```python
from build123d import *

# Parameters (mm, degrees)
SKETCH1_W           = 50.8
SKETCH1_H           = 50.8
BOSS_EXTRUDE1_DEPTH = 1.5875
SKETCH3_R           = 1.2065
BOSS_EXTRUDE2_DEPTH = 8.89
SKETCH4_R           = 2.54
SKETCH4_R_2         = 1.27
CUT_EXTRUDE1_DEPTH  = 43.790708396
BOSS_EXTRUDE3_START = 12.065
SKETCH5_R           = 1.2065
BOSS_EXTRUDE3_DEPTH = 12.065


with BuildPart() as part:
    # Sketch1 → Boss-Extrude1 (new, symmetric)
    with BuildSketch(Plane(origin=(0, 0, 0), x_dir=(1, 0, 0), z_dir=(0, 1, 0))):
        Rectangle(SKETCH1_W, SKETCH1_H)
    extrude(amount=BOSS_EXTRUDE1_DEPTH, both=True)

    # Sketch3 → Boss-Extrude2 (add)
    with BuildSketch(Plane(origin=(25.4, 0, 0), x_dir=(0, 0, -1), z_dir=(1, 0, 0))):
        with Locations(Location((0, 0, 0), (0, 0, 180))):
            Circle(SKETCH3_R)
    extrude(amount=BOSS_EXTRUDE2_DEPTH)

    # Sketch4 → Cut-Extrude1 (cut, through all)
    with BuildSketch(Plane(origin=(0, 1.5875, 0), x_dir=(1, 0, 0), z_dir=(0, 1, 0))):
        with Locations(Location((0, 0, 0), (0, 0, 270))):
            Circle(SKETCH4_R)
        with Locations(Location((-16.51, 16.51, 0), (0, 0, 270))):
            Circle(SKETCH4_R)
        with Locations(Location((16.51, 16.51, 0), (0, 0, 270))):
            Circle(SKETCH4_R)
        with Locations(Location((16.51, -16.51, 0), (0, 0, 270))):
            Circle(SKETCH4_R)
        with Locations(Location((-16.51, -16.51, 0), (0, 0, 270))):
            Circle(SKETCH4_R)
        with Locations(Location((-16.51, 7.62, 0), (0, 0, 270))):
            Circle(SKETCH4_R_2)
        with Locations(Location((-7.62, 16.51, 0), (0, 0, 270))):
            Circle(SKETCH4_R_2)
        with Locations(Location((7.62, 16.51, 0), (0, 0, 270))):
            Circle(SKETCH4_R_2)
        with Locations(Location((-16.51, -7.62, 0), (0, 0, 270))):
            Circle(SKETCH4_R_2)
        with Locations(Location((7.62, -16.51, 0), (0, 0, 90))):
            Circle(SKETCH4_R_2)
        with Locations(Location((-7.62, -16.51, 0), (0, 0, 90))):
            Circle(SKETCH4_R_2)
        with Locations(Location((16.51, -7.62, 0), (0, 0, 90))):
            Circle(SKETCH4_R_2)
        with Locations(Location((16.51, 7.62, 0), (0, 0, 90))):
            Circle(SKETCH4_R_2)
        with Locations(Location((5.578227154, 8.89, 0), (0, 0, 270))):
            Circle(SKETCH4_R_2)
        with Locations(Location((-5.578227154, 8.89, 0), (0, 0, 270))):
            Circle(SKETCH4_R_2)
        with Locations(Location((8.89, -5.578227154, 0), (0, 0, 270))):
            Circle(SKETCH4_R_2)
        with Locations(Location((8.89, 5.578227154, 0), (0, 0, 270))):
            Circle(SKETCH4_R_2)
        with Locations(Location((-5.578227154, -8.89, 0), (0, 0, 270))):
            Circle(SKETCH4_R_2)
        with Locations(Location((5.578227154, -8.89, 0), (0, 0, 270))):
            Circle(SKETCH4_R_2)
        with Locations(Location((-8.89, 5.578227154, 0), (0, 0, 270))):
            Circle(SKETCH4_R_2)
        with Locations(Location((-8.89, -5.578227154, 0), (0, 0, 270))):
            Circle(SKETCH4_R_2)
    extrude(amount=-CUT_EXTRUDE1_DEPTH, mode=Mode.SUBTRACT)

    # Sketch5 → Boss-Extrude3 (add)
    with BuildSketch(Plane.ZY.offset(25.4).offset(BOSS_EXTRUDE3_START)):
        Circle(SKETCH5_R)
    extrude(amount=-BOSS_EXTRUDE3_DEPTH)


solid = part.part
```
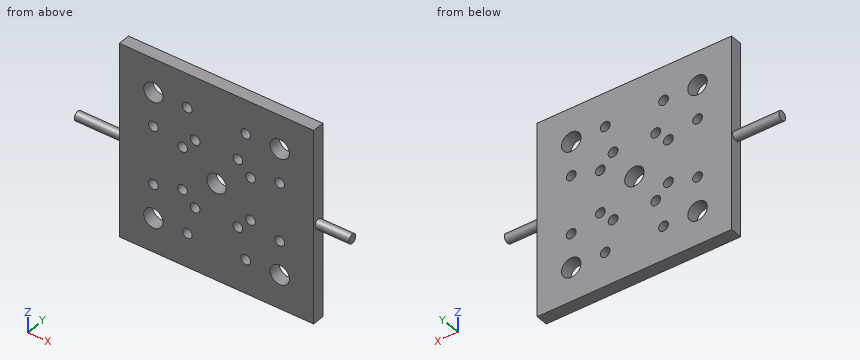
Can you work these out from the model? Positions are in its coordinate system, mm. Round coordinates to 2 decimals unless told otherwise and drop trailing zeros. Loops run counter-clockwise (first coordinate to the right, second up) from the corner with the lowest first, then second, coordinate; pieces in that order, holes last.
Item 1: Suppose I cut it at B-B, the plane z = -16.51. Write out the boundary of the cut face in (x, y), then the cut area to 3 significant figures.
Item 2: Please list where these lines run through material, in increasing order: L1, parallel to Z at x = 9, y = 1.4; L2, parallel to X at y = 0.35, z = -7.5; L3, parallel to Z at x = -14.5, y = -1.25.
Item 3: Will this pin go through, and if not, where does the flat tip stop? pin 1 Ø1 at (y, z) = (0.5, 9.5) entering from +X.
Item 4: Suppose I cut it at A-A, the plane x = 0. Write out the boundary of the cut face in (y, z), then the cut area to 3 significant figures.
Item 5: Suppose I cut it at D-D, the plane x = 16.51. Write out the boundary of the cut face in (y, z), then the cut area to 3 significant figures.
Reported:
1. outline: (-25.4, -1.59) - (-19.05, -1.59) - (-19.05, 1.59) - (-25.4, 1.59) - close; (-13.97, -1.59) - (-8.89, -1.59) - (-8.89, 1.59) - (-13.97, 1.59) - close; (-6.35, -1.59) - (6.35, -1.59) - (6.35, 1.59) - (-6.35, 1.59) - close; (8.89, -1.59) - (13.97, -1.59) - (13.97, 1.59) - (8.89, 1.59) - close; (19.05, -1.59) - (25.4, -1.59) - (25.4, 1.59) - (19.05, 1.59) - close
1. area: 113 mm2
2. L1: z = -25.4 to -6.84, -4.31 to 4.31, 6.84 to 25.4
2. L2: x = -25.4 to -17.77, -15.25 to 15.25, 17.77 to 25.4
2. L3: z = -25.4 to -18.06, -14.96 to 14.96, 18.06 to 25.4
3. pin 1: stops at x = 25.4
4. outline: (-1.59, -25.4) - (1.59, -25.4) - (1.59, -2.54) - (-1.59, -2.54) - close; (-1.59, 2.54) - (1.59, 2.54) - (1.59, 25.4) - (-1.59, 25.4) - close
4. area: 145 mm2
5. outline: (-1.59, -25.4) - (1.59, -25.4) - (1.59, -19.05) - (-1.59, -19.05) - close; (-1.59, -13.97) - (1.59, -13.97) - (1.59, -8.89) - (-1.59, -8.89) - close; (-1.59, -6.35) - (1.59, -6.35) - (1.59, 6.35) - (-1.59, 6.35) - close; (-1.59, 8.89) - (1.59, 8.89) - (1.59, 13.97) - (-1.59, 13.97) - close; (-1.59, 19.05) - (1.59, 19.05) - (1.59, 25.4) - (-1.59, 25.4) - close
5. area: 113 mm2
